Design review of the part built by this model. Coordinates are the model's own, in mm. A direction names the side the tool comes from. Give positions to 0.01 mm unless a question says otherwise; leave off trailing zeros. Loops run counter-clockwise (first coordinate to the right, second up) from the corner with the lowest first, then second, coordinate; pieces in that order, holes last. Notation, with made-up numbers: (77.5, 19) - (92.5, 19) arc R26 ccw to (92.5, 47) - close; hole circle Ø9 at (20.5, 85). An arc over 180 degrees is marked (long way). Put each result on its own line as item: value. Start each with the question number.
```python
from build123d import *

# Parameters (mm, degrees)
SKETCH1_W           = 85.725
SKETCH1_H           = 190.5
BOSS_EXTRUDE1_DEPTH = 3.175
SHELL1_T            = -1.27
FILLET1_R           = 3.175


with BuildPart() as part:
    # Sketch1 → Boss-Extrude1 (new body)
    with BuildSketch(Plane(origin=(0, 0, 0), x_dir=(1, 0, 0), z_dir=(0, 1, 0))):
        Rectangle(SKETCH1_W, SKETCH1_H)
    extrude(amount=BOSS_EXTRUDE1_DEPTH)

    # Shell1
    shell1_openings = [part.faces().sort_by_distance(p)[0] for p in [
        (0, 0, 0),
    ]]
    offset(amount=SHELL1_T, openings=shell1_openings, kind=Kind.INTERSECTION)

    # Fillet1
    fillet1_edges = [part.edges().sort_by_distance(p)[0] for p in [
        (-41.5925, 0.9525, -93.98),
        (-41.5925, 0.9525, 93.98),
        (41.5925, 0.9525, 93.98),
        (41.5925, 0.9525, -93.98),
    ]]
    fillet(fillet1_edges, radius=FILLET1_R)


solid = part.part
```
Item 1: Consider section C-C (x = 11). State the section outline as (y, z) points (3 decimals).
Item 2: Mouldability with a two-part tool opening along Z and no side actions: class faces 3 (the flat face through (-42.862, 2, 1)), 4 (the flat face through (-1, 2, -95.25)), 5 (the cylindrical face through (40.687, 0.939, -93.025)), 6 (the cylindrical face through (-40.687, 0.939, 93.025)) as pulls with the +Z half, pulls with the -Z half, needs draft (parallel to the pull), parting line crosses it, or undercut.
Item 3: For P1, Ø5, axis at x = 31.5, z = 50.5, coming from the -Y side (3 decimals), flat-tipped, find the tip position at first contact; note if it passes through.
Item 4: Machinability: for faces 1 (the flat face through (-1, 1.905, -1)), 2 (the flat face through (-1, 3.175, -1)), which of the approach directions +Z, -Z, +X, -X, +Y, -Y give a long, thin tool a straight path to every point of the face, cutting with its end or side? Answer none if there is none.
Item 5: For L1, parallel to X at y = 0.25, z = -16.5; L2, parallel to Z at x = 9, y = 0.45; L3, parallel to Y at x = 15.5, z = 2 (3 decimals), list the stretches that pass through material, from the lowest coordinate up. Write a range as from..to.
Item 6: Consider section B-B (z = 55). State the section outline as (x, y) points (1 decimal), plus the area to 3 significant figures.
Geometry says:
1. outline: (0, -95.25) - (3.175, -95.25) - (3.175, 95.25) - (0, 95.25) - (0, 93.98) - (1.905, 93.98) - (1.905, -93.98) - (0, -93.98) - close
2. face 3: needs draft
2. face 4: pulls with the -Z half
2. face 5: undercut
2. face 6: undercut
3. P1: stops at y = 1.905
4. face 1: -Y
4. face 2: +Z, -Z, +X, -X, +Y
5. L1: x = -42.86..-41.59, 41.59..42.86
5. L2: z = -95.25..-93.98, 93.98..95.25
5. L3: y = 1.905..3.175
6. outline: (-42.9, 0) - (-41.6, 0) - (-41.6, 1.9) - (41.6, 1.9) - (41.6, 0) - (42.9, 0) - (42.9, 3.2) - (-42.9, 3.2) - close
6. area: 114 mm2
